Here's the drawing with two shaded views (mm, measured from the low corner). I have some questions. A direction names the side the tool comes from. Coordinates: 2 decimals unless noted, no trailing zeros. Order: outer loops, then holes, each group sorted by start corner. A loop starts at its lowest first (then second) coordinate and runs counter-clockwise, first axis right, second up. Notation, with made-up numbers: (-18, 76) - (-5, 76) arc R19 cw to (-5, 94) - close; hole circle Ø5 at (-9.75, 84). An arc over 180 degrees is marked (long way). Answer as a JSON object with one key per item and string values. Group by question number.
(1) Imagine slicing it at D-D, the plane x = 15. Write out the boundary of the cut face in (y, z).
(2) Please list where these lines run through material, in increasing order: probe 1 along Z at (x, y) = (8.5, 0.7); probe 2 along X at (y, z) = (3.45, 10); probe 3 along Y at (x, z) = (13.75, 1.5).
(3) Will these pins go through, and if not, where does the flat tip stop? P1, Ø3, axis at x = 8.5, z = 3, coming from the +Y side; P2, Ø0.8, axis at y = 3.5, z = 5, coming from the +X side; P3, Ø5, axis at x = 15, z = 6.5, coming from the +Y side; P4, Ø0.6, axis at x = 2.5, y = 3, coming from the -Z side.
(4) We'd pull the mould along X, two halves only. Please class the marked faces 5, 6 and 7: pulls with the +X half, pulls with the -X half, needs draft (parallel to the pull), parting line crosses it, or undercut.
(5) Imagine slicing it at B-B, the plane y = 3.7. Write out the boundary of the cut face in (x, z), and give its area (3 significant figures).
(6) Imagine slicing it at C-C, the plane z = 3. Write out the boundary of the cut face in (x, y), and give its area (3 significant figures).
(7) Imagine slicing it at A-A, the plane x = 8.5. Write out the boundary of the cut face in (y, z).
(8) Which directions (+Z, -Z, +X, -X, +Y, -Y) give clear straight access to the entire face, cutting with the end or side of a thin tool? Please do the marked faces 1, 2, 3 and 4.
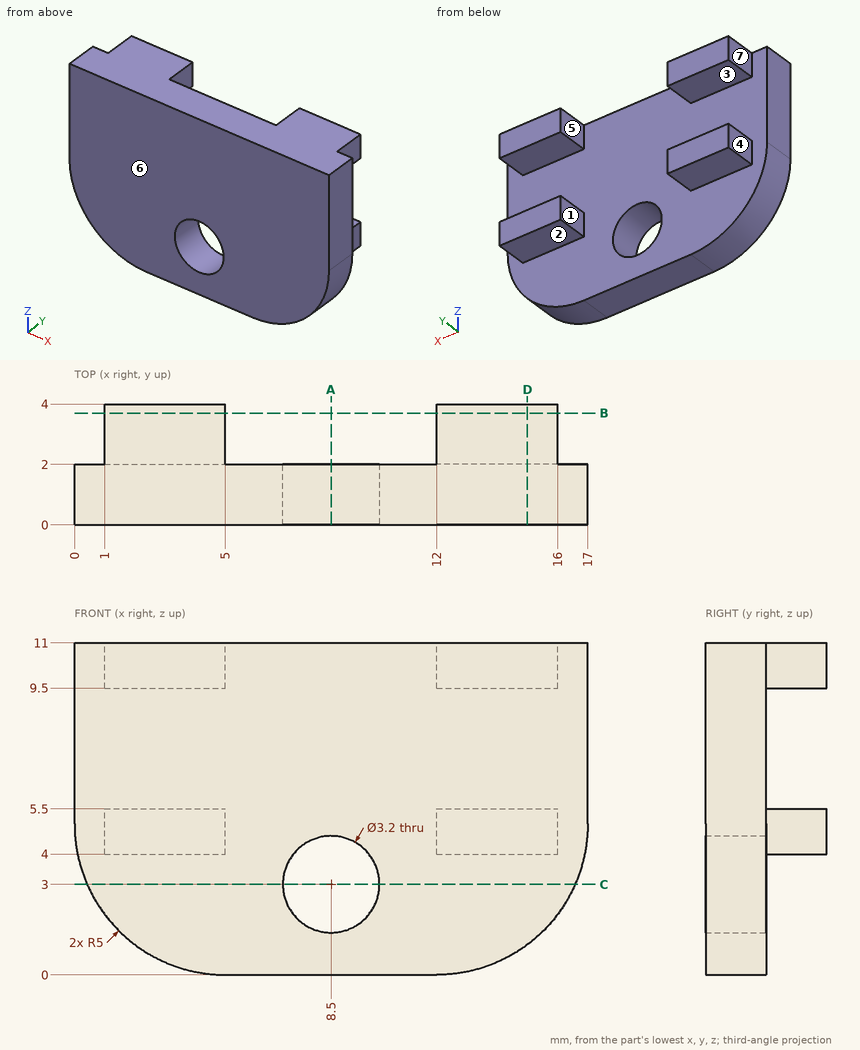
Result set:
{
 "1": {"outline": "(0, 1) - (2, 1) - (2, 4) - (4, 4) - (4, 5.5) - (2, 5.5) - (2, 9.5) - (4, 9.5) - (4, 11) - (0, 11) - close"},
 "2": {"probe 1": "z = 0 to 1.4, 4.6 to 11", "probe 2": "x = 1 to 5, 12 to 16", "probe 3": "y = 0 to 2"},
 "3": {"P1": "passes through", "P2": "stops at x = 16", "P3": "stops at y = 4", "P4": "stops at z = 4"},
 "4": {"face 5": "undercut", "face 6": "needs draft", "face 7": "pulls with the -X half"},
 "5": {"outline": "(1, 4) - (5, 4) - (5, 5.5) - (1, 5.5) - close; (1, 9.5) - (5, 9.5) - (5, 11) - (1, 11) - close; (12, 4) - (16, 4) - (16, 5.5) - (12, 5.5) - close; (12, 9.5) - (16, 9.5) - (16, 11) - (12, 11) - close", "area": "24.0 mm^2"},
 "6": {"outline": "(0.42, 0) - (6.9, 0) - (6.9, 2) - (0.42, 2) - close; (10.1, 0) - (16.58, 0) - (16.58, 2) - (10.1, 2) - close", "area": "25.9 mm^2"},
 "7": {"outline": "(0, 0) - (2, 0) - (2, 1.4) - (0, 1.4) - close; (0, 4.6) - (2, 4.6) - (2, 11) - (0, 11) - close"},
 "8": {"face 1": "+Z, -Z, +Y", "face 2": "-Z, +X, -X, +Y", "face 3": "+X, -X, +Y", "face 4": "+Z, -Z, -X, +Y"}
}
